For this review, take the finished solid that the model builds, in its own axes (mm). A direction names the side the tool comes from. Round coordinates to 2 decimals unless told otherwise and drop trailing zeros. Loops run counter-clockwise (first coordinate to the right, second up) from the corner with the lowest first, then second, coordinate; pieces in that order, holes last. Notation, with made-up numbers: (20.5, 58) -> (75.5, 58) arc R32 cw to (75.5, 84) -> close; hole circle Ø11 at (55.5, 28). An arc over 180 degrees is marked (long way). Write each question's results on one line, items separated by ' | '.
```python
from build123d import *

# Parameters (mm, degrees)
PAD_DEPTH       = 80
SKETCH001_W     = 25
SKETCH001_H     = 30
SKETCH001_R     = 3.25
POCKET_DEPTH    = 45.001
FILLET_R        = 0.8
SKETCH002_W     = 52
SKETCH002_H     = 37
POCKET001_DEPTH = 8
FILLET001_R     = 0.8
FILLET002_R     = 0.8


with BuildPart() as part:
    # Sketch → Pad (new body)
    with BuildSketch(Plane.XZ):
        with BuildLine():
            Line((-15, 10), (15, 10))
            Line((15, 10), (15, 0.75))
            Line((15, 0.75), (5, 0.75))
            ThreePointArc((5, 0.75), (-7.454837, 0), (5, -0.75))
            Line((15, -0.75), (5, -0.75))
            Line((15, -10), (15, -0.75))
            Line((15, -10), (-15, -10))
            Line((-15, -22.5), (-15, -10))
            Line((-75, -22.5), (-15, -22.5))
            Line((-75, 22.5), (-75, -22.5))
            Line((-15, 22.5), (-75, 22.5))
            Line((-15, 10), (-15, 22.5))
        make_face()
    extrude(amount=PAD_DEPTH)

    # Sketch001 (on Face9 of Pad) → Pocket (cut, through all)
    with BuildSketch(Plane(origin=(0, 0, -22.5), x_dir=(1, 0, 0), z_dir=(0, 0, -1))):
        with Locations((2.5, 40)):
            Rectangle(SKETCH001_W, SKETCH001_H)
        with BuildLine():
            Line((-20, 80), (-75, 80))
            Line((-75, 80), (-75, 10))
            add(Edge.make_bspline(
                [(-75, 10), (-40, 16), (-20, 80)],
                knots=[0, 0, 0, 1, 1, 1], degree=2))
        make_face()
        with Locations((10, 12.5)):
            Circle(SKETCH001_R)
        with Locations((10, 67.5)):
            Circle(SKETCH001_R)
    extrude(amount=-POCKET_DEPTH, mode=Mode.SUBTRACT)

    # Fillet
    fillet_edges = [part.edges().sort_by_distance(p)[0] for p in [
        (-38.841084, -37.393675, -22.5),
        (-20, -80, 0),
        (-38.841077, -37.393686, 22.5),
        (-75, -10, 0),
    ]]
    fillet(fillet_edges, radius=FILLET_R)

    # Sketch002 (on Face17 of Fillet) → Pocket001 (cut)
    with BuildSketch(Plane(origin=(0, 0, 0), x_dir=(1, 0, 0), z_dir=(0, 1, 0))):
        with Locations((-45, 0)):
            Rectangle(SKETCH002_W, SKETCH002_H)
    extrude(amount=-POCKET001_DEPTH, mode=Mode.SUBTRACT)

    # Fillet001
    fillet001_edges = [part.edges().sort_by_distance(p)[0] for p in [
        (15, 0, 5.375),
        (15, -12.5, 0.75),
        (15, -25, 5.375),
        (15, -12.5, 10),
        (15, 0, -5.375),
        (15, -12.5, -0.75),
        (15, -25, -5.375),
        (15, -12.5, -10),
        (15, -55, 5.375),
        (15, -67.5, 0.75),
        (15, -80, 5.375),
        (15, -67.5, 10),
        (15, -55, -5.375),
        (15, -67.5, -0.75),
        (15, -80, -5.375),
        (15, -67.5, -10),
    ]]
    fillet(fillet001_edges, radius=FILLET001_R)

    # Fillet002
    fillet002_edges = [part.edges().sort_by_distance(p)[0] for p in [
        (-15, -40, 22.5),
        (-15, -80, 16.25),
        (-15, -80, -16.25),
        (-15, -40, -22.5),
    ]]
    fillet(fillet002_edges, radius=FILLET002_R)


solid = part.part
```
1. Consider section B-B (y = -4.5). State the section outline as (x, z) points, plus the area to 3 significant figures.
Values found:
outline: (-75, -22.5) -> (-15.8, -22.5) arc R0.8 ccw to (-15, -21.7) -> (-15, -10) -> (14.2, -10) arc R0.8 ccw to (15, -9.2) -> (15, -1.55) arc R0.8 ccw to (14.2, -0.75) -> (5, -0.75) arc R6.25 cw (long way) to (5, 0.75) -> (14.2, 0.75) arc R0.8 ccw to (15, 1.55) -> (15, 9.2) arc R0.8 ccw to (14.2, 10) -> (-15, 10) -> (-15, 21.7) arc R0.8 ccw to (-15.8, 22.5) -> (-75, 22.5) -> close; hole (-71, -18.5) -> (-19, -18.5) -> (-19, 18.5) -> (-71, 18.5) -> close | area: 1,240 mm2
2. To check wall thickness, follow probe 1 along Y at (x, z) = (10, 4); probe 2 along Y at (x, z) = (-4, 8); probe 3 along X at (y, z) = (-65, 5.5). State the ranges of each line that lie inside material, in increasing order.
Values found:
probe 1: y = -80 to -70.75, -64.25 to -55, -25 to -15.75, -9.25 to 0 | probe 2: y = -80 to -55, -25 to 0 | probe 3: x = -25.2 to -4.17, 1.76 to 7.92, 12.08 to 15
3. For pin 1 (4 mm diameter, centred on x = 10, y = -12.5, fed in from -Z); pin 2 (7.5 mm diameter, centred on x = 8, y = -11.5, fed in from -Z); pin 3 (6 mm diameter, centred on y = -55.5, z = 13.5, fed in from +X); pin 4 (11 mm diameter, centred on x = -33.5, z = -5.5, fed in from +Y), all flat-tipped, find the tip position at first contact; note any pin that passes through.
Values found:
pin 1: passes through | pin 2: stops at z = -10 | pin 3: stops at x = -15 | pin 4: stops at y = -8
4. Tool access review of faces 1 (the face through (-15, -39, 16)), 2 (the face through (6.6, -12.3, -0.75)), 3 (the face through (-15, -39, -16)): name each direction out of +Z, -Z, +X, -X, +Y, -Y from which nothing blocks a thin tool from reaching the whole face with its end or side.
Values found:
face 1: +Z, +X, +Y, -Y | face 2: +X, +Y, -Y | face 3: -Z, +X, +Y, -Y
5. Consider section A-A (x = 10). Give the number of separate pieces and of enclosed holes in the cut face, plus the area to 4 significant figures.
Values found:
separate pieces: 8 | enclosed holes: 0 | area: 684.5 mm2
6. Consider section C-C (x = -12). State the section outline as (y, z) points, plus the area to 3 significant figures.
Values found:
outline: (-80, -10) -> (0, -10) -> (0, 10) -> (-80, 10) -> close | area: 1,600 mm2
7. Draft analysis for pull direction X (two halves, no side actions). For faces 4 (the face through (15, -12, -5)), 5 (the face through (6.753, -12.643, 5.31)), 6 (the face through (-11, -39, 10)), state which applies: released by +X, released by -X, zero draft, split by the parting line, or undercut.
Values found:
face 4: released by +X | face 5: undercut | face 6: zero draft
